```python
from build123d import *

# Parameters (mm, degrees)
BOSS_EXTRUDE2_DEPTH = 410
FILLET1_R           = 10
FILLET2_R           = 5


with BuildPart() as part:
    # Sketch1 → Boss-Extrude2 (new body)
    with BuildSketch(Plane(origin=(0, 0, 0), x_dir=(1, 0, 0), z_dir=(0, 1, 0))):
        Polygon((-113.923660484, 64.911766887), (-73.923660484, 64.911766887), (-69.59269291, 79.161766887), (-67.59269291, 79.161766887), (-67.59269291, 93.411766887), (-64.59269291, 93.411766887), (-64.59269291, 28.411766887), (-67.59269291, 28.411766887), (-67.59269291, 42.661766887), (-69.59269291, 42.661766887), (-73.923660484, 56.911766887), (-113.923660484, 56.911766887), (-113.923660484, 28.411766887), (-117.923660484, 28.411766887), (-117.923660484, 93.411766887), (-113.923660484, 93.411766887), align=None)
    extrude(amount=BOSS_EXTRUDE2_DEPTH)

    # Fillet1
    # the kernel refuses this fillet: 10 mm, written as the material it takes off along each edge
    with BuildSketch(Plane(origin=(-113.923660484, -20, -93.411766887), x_dir=(-1, 0, 0), z_dir=(0, 1, 0))) as fillet1_piece_1:
        with BuildLine():
            CenterArc((10, 8), FILLET1_R, 180, 53.130102354)
            Line((0, 8), (-0.2, 8))
            Line((-0.2, 8), (-0.2, 0))
            Line((-0.2, 0), (0, -0.2))
            ThreePointArc((0, -0.2), (2, -0.2), (3.88, -0.16))
            Line((3.88, -0.16), (4, 0))
        make_face()
    extrude(amount=450, mode=Mode.SUBTRACT)
    with BuildSketch(Plane(origin=(-113.923660484, -20, -28.411766887), x_dir=(0, 0, -1), z_dir=(0, 1, 0))) as fillet1_piece_2:
        with BuildLine():
            CenterArc((8, 10), FILLET1_R, 216.869897646, 53.130102354)
            Line((0, 4), (-0.16, 3.88))
            ThreePointArc((-0.16, 3.88), (-0.2, 2), (-0.2, 0))
            Line((-0.2, 0), (0, -0.2))
            Line((0, -0.2), (8, -0.2))
            Line((8, -0.2), (8, 0))
        make_face()
    extrude(amount=450, mode=Mode.SUBTRACT)

    # Fillet2
    fillet2_edges = [part.edges().sort_by_distance(p)[0] for p in [
        (-113.923660484, 205, -64.911766887),
        (-73.923660484, 205, -64.911766887),
        (-73.923660484, 205, -56.911766887),
        (-113.923660484, 205, -56.911766887),
    ]]
    fillet(fillet2_edges, radius=FILLET2_R)


solid = part.part
```
Geometry: final body of the model. Coordinates: model frame, mm. A direction names the side the tool comes from. Give positions to 0.01 mm unless a question says otherwise; leave off trailing zeros. Loops run counter-clockwise (first coordinate to the right, second up) from the corner with the lowest first, then second, coordinate; pieces in that order, holes last. Notation, with made-up numbers: (57.25, 53) -> (68.25, 53) arc R8 ccw to (68.25, 57) -> close; hole circle Ø4 at (53.25, -8.75). An arc over 180 degrees is marked (long way). Use one line per item in the form item = value.
Item 1: Line query: probe 1 along X at (y, z) = (83.5, -40.5); probe 2 along Z at (x, y) = (-86.5, 324.5); probe 3 along X at (y, z) = (34.5, -73.5). Output: solid intervals per line, ascending.
A:
probe_1 = -117.92 to -113.92, -67.59 to -64.59
probe_2 = -64.91 to -56.91
probe_3 = -117.92 to -113.92, -71.31 to -64.59
Item 2: Section query B-B on x = -93.5. Output: boundary loops of the cut face in (y, z), and give its area (3 significant figures).
A:
outline = (0, -64.91) -> (410, -64.91) -> (410, -56.91) -> (0, -56.91) -> close
area = 3,280 mm^2
Item 3: Pin query (flat end, axial travel): P1, Ø2, axis at x = -105, y = 314, coming from the -Z side; P2, Ø2, axis at x = -69, y = 234, coming from the +Z side; P3, Ø0.6, axis at x = -69, y = 164.5, coming from the -Z side; P4, Ø8, axis at x = -71.5, y = 309.5, coming from the -Z side. Return the tip coordinate at first contact, or that it passes through.
A:
P1 = -64.91
P2 = -42.66
P3 = -79.16
P4 = -93.41
Item 4: Draft query along X for faces 1 (the face through (-64.593, 202, -61)), 2 (the face through (-93, 202, -64.912)), 3 (the face through (-117.924, 202, -60)). Return one class per face: pulls with the +X half, pulls with the -X half, needs draft (parallel to the pull), parting line crosses it, or undercut.
A:
face_1 = pulls with the +X half
face_2 = undercut
face_3 = pulls with the -X half
Item 5: Section query A-A on y = 339. Output: boundary loops of the cut face in (x, z), and give its area (3 significant figures).
A:
outline = (-117.92, -93.41) arc R10 ccw to (-113.92, -85.41) -> (-113.92, -69.91) arc R5 cw to (-108.92, -64.91) -> (-77.63, -64.91) arc R5 cw to (-72.85, -68.46) -> (-69.59, -79.16) -> (-67.59, -79.16) -> (-67.59, -93.41) -> (-64.59, -93.41) -> (-64.59, -28.41) -> (-67.59, -28.41) -> (-67.59, -42.66) -> (-69.59, -42.66) -> (-72.85, -53.37) arc R5 cw to (-77.63, -56.91) -> (-108.92, -56.91) arc R5 cw to (-113.92, -51.91) -> (-113.92, -36.41) arc R10 ccw to (-117.92, -28.41) -> close
area = 941 mm^2
Item 6: Access query for faces 4 (the face through (-89, 410, -61)), 5 (the face through (-67.593, 202, -86)), 6 (the face through (-67.593, 202, -35)). Directions: +Z, -Z, +X, -X, +Y, -Y. A direction counts if a zero-diameter tool reaches every point of the face in a straight line with its end or side. Return the directions, or none.
A:
face_4 = +Z, -Z, +X, -X, +Y
face_5 = -Z, +Y, -Y
face_6 = +Z, +Y, -Y
